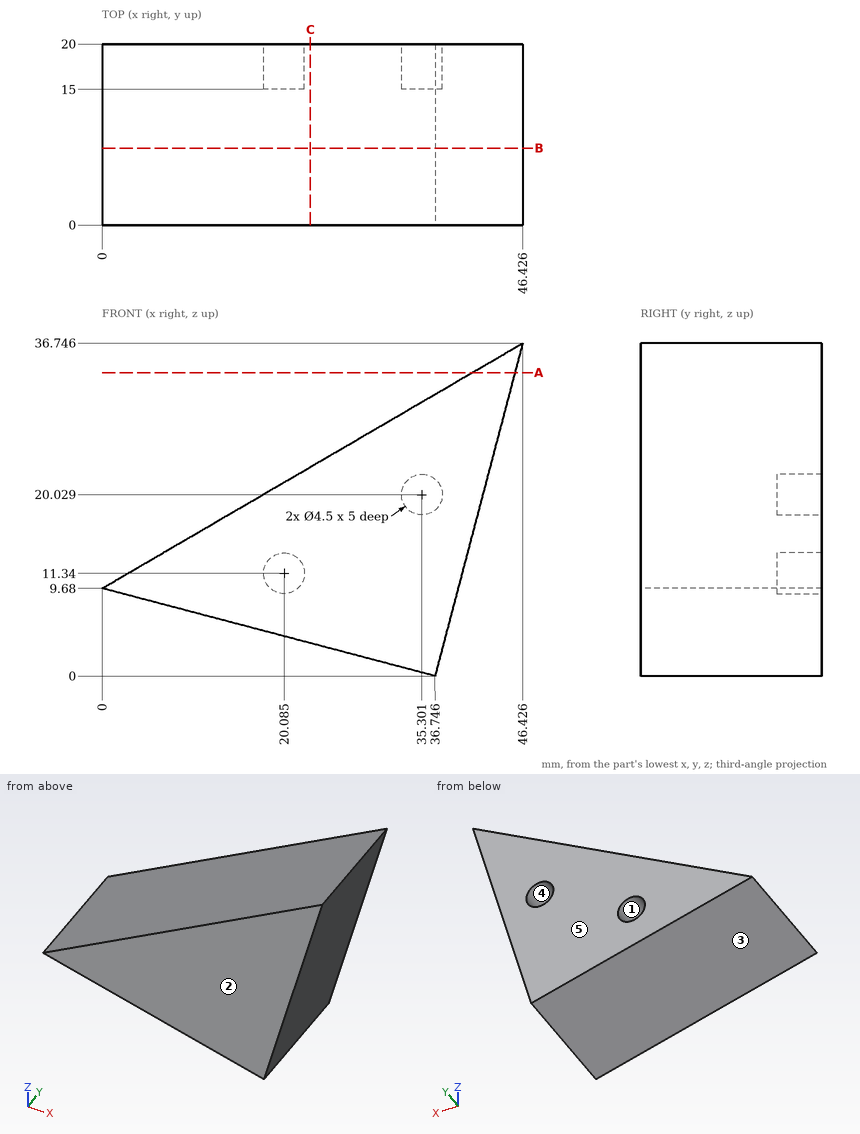
Job drawing, mm, ordinate dimensions from the low corner. One solid piece. A direction names the side the tool comes from. Coordinates: 2 decimals unless noted, no trailing zeros. Loops run counter-clockwise (first coordinate to the right, second up) from the corner with the lowest first, then second, coordinate; pieces in that order, holes last. Notation, with made-up numbers: (34, 46) -> (88, 46) arc R29 cw to (88, 77) -> close; hole circle Ø8 at (88, -8). An arc over 180 degrees is marked (long way). One line per item, written item: value.
1. Slice it at B-B on y = 8.5. Write the cut outline in (x, z), and give its area (3 significant figures).
Answers:
outline: (0, 9.68) -> (36.75, 0) -> (46.43, 36.75) -> close
area: 722 mm^2
2. Which spindle directions (+Z, -Z, +X, -X, +Y, -Y) get a long thin tool onto all of the face, cutting with end or side? Do the marked faces 4 and 5. Say none if no direction does.
Answers:
face 4: +Y
face 5: +Z, -Z, +X, -X, +Y
3. Slice it at C-C on x = 23. Write the cut outline in (y, z).
Answers:
outline: (0, 3.62) -> (20, 3.62) -> (20, 23.09) -> (0, 23.09) -> close
4. Flat gauge pins, fed straight in: P1, Ø5, axis at x = 41.5, y = 13, coming from the +Z side; P2, Ø5, axis at x = 22.5, y = 17.5, coming from the -Z side (1 decimal); P3, Ø1.3, axis at x = 19.5, z = 11, coming from the +Y side. Where does each tip first touch, or does it go through?
Answers:
P1: stops at z = 35.33
P2: stops at z = 3.1
P3: stops at y = 15
5. Slice it at A-A on z = 33.5. Write the cut outline in (x, y).
Answers:
outline: (40.86, 0) -> (45.57, 0) -> (45.57, 20) -> (40.86, 20) -> close
6. Drill centre lines: line 1 (X direction, y = 3.5, z = 18.5) (1 decimal); line 2 (X direction, y = 12, z = 14.5) (1 decimal); line 3 (X direction, y = 18.5, z = 13) (1 decimal). Where is each one in solid material? Low to high. Write a range as [from, to].
Answers:
line 1: x = [15.1, 41.6]
line 2: x = [8.3, 40.6]
line 3: x = [5.7, 18.6], [21.6, 40.2]
7. Pull direction Z, two halves, no side cores. Call the marked faces 1, 2 and 3: pulls with the +Z half, pulls with the -Z half, needs draft (parallel to the pull), parting line crosses it, or undercut.
Answers:
face 1: undercut
face 2: needs draft
face 3: pulls with the -Z half
